Geometry check sheet. Reference: the model listing, model coordinates, mm. A direction names the side the tool comes from. Give positions to 0.01 mm unless a question says otherwise; leave off trailing zeros. Write each loop counter-clockwise with the first axis right and the second up, starting at its lowest first coordinate (ties: lowest second). Pieces come first, ordered by that corner, then holes.
(1) Cross-section at B-B (x = 0). Record the boundary of the cut face in (y, z), and give its area (3 significant figures).
(2) Thickness scan on line 1 along Y through (x, z) = (0, 0.45); line 2 along Y through (x, z) = (0, 4.75); line 3 along X through (y, z) = (-30.5, 2.25). Record the ranges inside material, lowest first.
(3) Cross-section at A-A (y = -41.5). Record the boundary of the cut face in (x, z).
(4) Mould release check, pull along X, two halves, no side actions. Record for faces 1 (the cylindrical face through (0, -75, 3)), 2 (the cylindrical face through (0, -43, 3)), 3 (the flat face through (-10, -1, 3)): +X half, -X half, draft (parallel to the pull), parting line (faces both ways), or undercut.
(5) Depth check by flat-ended pin: P1, Ø1.8, axis at x = 0, y = -18.5, coming from the +Z side. Enter the tip coordinate at first touch or a pass-through.
(6) Tool access check on faces 4 (the flat face through (3, 62, 0.95)), 5 (the cylindrical face through (8.112, 66.265, 2.369)), 6 (the cylindrical face through (-0.48, 68.62, 0.48)). Record the directions out of +Z, -Z, +X, -X, +Y, -Y that give a thin tool (end or side, any length) a straight path to the whole face; none if there is none.
```python
from build123d import *

# Parameters (mm, degrees)
SALIENTE_EXTRUIR1_DEPTH = 6.35
CROQUIS2_R              = 6.35
CORTAR_EXTRUIR1_DEPTH   = 5.4
CROQUIS3_R              = 3.65
CORTAR_EXTRUIR2_DEPTH   = 5.4
CROQUIS4_R              = 5
CROQUIS4_R_2            = 1.5
CORTAR_EXTRUIR3_DEPTH   = 7.35
CROQUIS5_R              = 1.5
CORTAR_EXTRUIR4_DEPTH   = 10


with BuildPart() as part:
    # Croquis1 → Saliente-Extruir1 (new body)
    with BuildSketch(Plane.XY):
        with BuildLine():
            Line((10, 65), (10, -65))
            ThreePointArc((10, -65), (0, -75), (-10, -65))
            Line((-10, -65), (-10, 65))
            ThreePointArc((-10, 65), (0, 75), (10, 65))
        make_face()
    extrude(amount=SALIENTE_EXTRUIR1_DEPTH)

    # Croquis2 → Cortar-Extruir1 (cut)
    with BuildSketch(Plane.XY.offset(6.35)):
        with Locations((0, 65)):
            Circle(CROQUIS2_R)
    extrude(amount=-CORTAR_EXTRUIR1_DEPTH, mode=Mode.SUBTRACT)

    # Croquis3 → Cortar-Extruir2 (cut)
    with BuildSketch(Plane.XY.offset(0.95)):
        with Locations((0, 65)):
            Circle(CROQUIS3_R)
    extrude(amount=-CORTAR_EXTRUIR2_DEPTH, mode=Mode.SUBTRACT)

    # Croquis4 → Cortar-Extruir3 (cut, through all)
    with BuildSketch(Plane.XY.offset(6.35)):
        with Locations((0, -30)):
            Circle(CROQUIS4_R)
        with Locations((0, -18.5)):
            Circle(CROQUIS4_R_2)
        with Locations((0, -41.5)):
            Circle(CROQUIS4_R_2)
    extrude(amount=-CORTAR_EXTRUIR3_DEPTH, mode=Mode.SUBTRACT)

    # Croquis5 → Cortar-Extruir4 (cut)
    with BuildSketch(Plane(origin=(10, 0, 0), x_dir=(0, 0, -1), z_dir=(1, 0, 0))):
        with Locations((-3.175, 65)):
            Circle(CROQUIS5_R)
    extrude(amount=-CORTAR_EXTRUIR4_DEPTH, mode=Mode.SUBTRACT)


solid = part.part
```
Reply:
1. outline: (-75, 0) - (-43, 0) - (-43, 6.35) - (-75, 6.35) - close; (-40, 0) - (-35, 0) - (-35, 6.35) - (-40, 6.35) - close; (-25, 0) - (-20, 0) - (-20, 6.35) - (-25, 6.35) - close; (-17, 0) - (61.35, 0) - (61.35, 0.95) - (58.65, 0.95) - (58.65, 6.35) - (-17, 6.35) - close; (68.65, 0) - (75, 0) - (75, 6.35) - (71.35, 6.35) - (71.35, 0.95) - (68.65, 0.95) - close
1. area: 775 mm2
2. line 1: y = -75 to -43, -40 to -35, -25 to -20, -17 to 61.35, 68.65 to 75
2. line 2: y = -75 to -43, -40 to -35, -25 to -20, -17 to 58.65, 71.35 to 75
2. line 3: x = -10 to -4.97, 4.97 to 10
3. outline: (-10, 0) - (-1.5, 0) - (-1.5, 6.35) - (-10, 6.35) - close; (1.5, 0) - (10, 0) - (10, 6.35) - (1.5, 6.35) - close
4. face 1: parting line
4. face 2: undercut
4. face 3: -X half
5. P1: passes through
6. face 4: +Z
6. face 5: +X
6. face 6: +Z, -Z
